Design review of the part built by this model. Coordinates are the model's own, in mm. A direction names the side the tool comes from. Coordinates: 2 decimals unless noted, no trailing zeros. Loops run counter-clockwise (first coordinate to the right, second up) from the corner with the lowest first, then second, coordinate; pieces in that order, holes last. Notation, with made-up numbers: M 37,-35 L 94,-35 A21 cw 94,-8 Z; hole C 10,47.25 d5. An arc over 180 degrees is marked long. Answer as a JSON object with one key per item and string values. Group by question number.
1. Draft analysis for pull direction Y (two halves, no side actions). For faces 1 (the cylindrical face through (11.27, 9.34, 7.3)), 2 (the cylindrical face through (1.7, 20.4, -2.2)), 3 (the cylindrical face through (4.054, 1.451, -3.168)), state which applies: +Y half, -Y half, draft (parallel to the pull), parting line (faces both ways), or undercut.
2. Insertion check: pin 1 (2 mm diameter, centred on x = 5.5, z = -2.5, fed in from -Y); pin 2 (1.8 mm diameter, centred on x = 10.5, y = 9.5, fed in from -Z); pin 3 (5.5 mm diameter, centred on x = 5.5, z = -3.5, fed in from +Y); pin 4 (1.5 mm diameter, centred on y = 3, z = 28, fed in from -X). Each pin has a flat end and moves straight along its axis. Give the tip position at first contact, or say it passes through.
3. Consider section C-C (x = 5.1). State the section outline as (y, z) points, then the cut area to 3 significant figures.
4. To check wall thickness, follow probe 1 along Z at (x, y) = (1.75, 19); probe 2 along Z at (x, y) = (1.75, 5.5); probe 3 along Y at (x, z) = (9.25, 13). State the ranges of each line that lie inside material, in increasing order.
5. Machinability: for faces 4 (the flat face through (6, 10, -0.9)), 5 (the cylindrical face through (0.63, 9.34, 7.3)), 6 (the flat face through (11.4, 0.5, 14.4)), 7 (the flat face through (6, 18.4, -2)), 8 (the cylindrical face through (0.66, 0.63, -0.46)), which of the approach directions +Z, -Z, +X, -X, +Y, -Y give a long, thin tool a straight path to every point of the face, cutting with its end or side? Answer none if there is none.
6. Consider section D-D (y = 5). State the section outline as (x, z) points, then the cut area to 3 significant figures.
7. Consider section B-B (y = 19). State the section outline as (x, z) points.
from build123d import *

# Parameters (mm, degrees)
SKETCH3_W           = 11.9
SKETCH3_H           = 10
BOSS_EXTRUDE1_DEPTH = 14.4
FILLET6_R           = 2.2
SKETCH6_W           = 11.9
SKETCH6_H           = 10
BOSS_EXTRUDE2_DEPTH = 8.9
SKETCH7_R           = 1.45
BOSS_EXTRUDE3_DEPTH = 9.5
SKETCH8_W           = 11.9
SKETCH8_H           = 18.4
BOSS_EXTRUDE4_DEPTH = 0.9
FILLET7_R           = 2.2
SKETCH9_R           = 4
BOSS_EXTRUDE6_DEPTH = 4.6
SKETCH10_W          = 11.9
SKETCH10_H          = 4.4
BOSS_EXTRUDE7_DEPTH = 4
SKETCH11_R          = 0.7
SKETCH11_R_2        = 0.702469816
SKETCH11_R_3        = 0.700963309
BOSS_EXTRUDE8_DEPTH = 4


with BuildPart() as part:
    # Sketch3 → Boss-Extrude1 (new body)
    with BuildSketch(Plane.XY):
        with Locations((5.95, 5)):
            Rectangle(SKETCH3_W, SKETCH3_H)
    extrude(amount=BOSS_EXTRUDE1_DEPTH)

    # Fillet6
    fillet6_edges = [part.edges().sort_by_distance(p)[0] for p in [
        (0, 10, 7.2),
        (11.9, 10, 7.2),
        (11.9, 0, 7.2),
        (0, 0, 7.2),
    ]]
    fillet(fillet6_edges, radius=FILLET6_R)

    # Sketch6 → Boss-Extrude2 (add)
    with BuildSketch(Plane.XY.offset(14.4)):
        with Locations((5.95, 5)):
            Rectangle(SKETCH6_W, SKETCH6_H)
    extrude(amount=BOSS_EXTRUDE2_DEPTH)

    # Sketch7 → Boss-Extrude3 (add)
    with BuildSketch(Plane.XY.offset(23.3)):
        with Locations((6.035152891, 5)):
            Circle(SKETCH7_R)
    extrude(amount=BOSS_EXTRUDE3_DEPTH)

    # Sketch8 → Boss-Extrude4 (add)
    with BuildSketch(Plane(origin=(0, 0, 0), x_dir=(-1, 0, 0), z_dir=(0, 0, -1))):
        with Locations((-5.95, 9.2)):
            Rectangle(SKETCH8_W, SKETCH8_H)
    extrude(amount=BOSS_EXTRUDE4_DEPTH)

    # Fillet7
    fillet7_edges = [part.edges().sort_by_distance(p)[0] for p in [
        (0, 0, -0.45),
        (11.9, 0, -0.45),
    ]]
    fillet(fillet7_edges, radius=FILLET7_R)

    # Sketch9 → Boss-Extrude6 (add)
    with BuildSketch(Plane(origin=(0, 0, -0.9), x_dir=(-1, 0, 0), z_dir=(0, 0, -1))):
        with Locations((-5.9, 5)):
            Circle(SKETCH9_R)
    extrude(amount=BOSS_EXTRUDE6_DEPTH)

    # Sketch10 → Boss-Extrude7 (add)
    with BuildSketch(Plane(origin=(0, 0, -0.9), x_dir=(-1, 0, 0), z_dir=(0, 0, -1))):
        with Locations((-5.95, 16.2)):
            Rectangle(SKETCH10_W, SKETCH10_H)
    extrude(amount=BOSS_EXTRUDE7_DEPTH)

    # Sketch11 → Boss-Extrude8 (add)
    with BuildSketch(Plane(origin=(0, 18.4, 0), x_dir=(1, 0, 0), z_dir=(0, 1, 0))):
        with Locations(Location((3.4, 2.9, 0), (0, 0, 90))):
            Circle(SKETCH11_R)
        with Locations(Location((5.1, 2.9, 0), (0, 0, 90))):
            Circle(SKETCH11_R)
        with Locations(Location((6.8, 2.9, 0), (0, 0, 90))):
            Circle(SKETCH11_R)
        with Locations(Location((8.5, 2.9, 0), (0, 0, 90))):
            Circle(SKETCH11_R_2)
        with Locations(Location((10.2, 2.9, 0), (0, 0, 90))):
            Circle(SKETCH11_R_3)
        with Locations(Location((1.7, 2.9, 0), (0, 0, 90))):
            Circle(SKETCH11_R)
    extrude(amount=BOSS_EXTRUDE8_DEPTH)


solid = part.part
Findings below:
{
 "1": {"face 1": "+Y half", "face 2": "draft", "face 3": "undercut"},
 "2": {"pin 1": "stops at y = 1", "pin 2": "stops at z = -0.9", "pin 3": "stops at y = 22.4", "pin 4": "stops at x = 5.3"},
 "3": {"outline": "M 0,-0.9 L 1.08,-0.9 L 1.08,-5.5 L 8.92,-5.5 L 8.92,-0.9 L 14,-0.9 L 14,-4.9 L 18.4,-4.9 L 18.4,-3.6 L 22.4,-3.6 L 22.4,-2.2 L 18.4,-2.2 L 18.4,0 L 10,0 L 10,23.3 L 6.11,23.3 L 6.11,32.8 L 3.89,32.8 L 3.89,23.3 L 0,23.3 Z", "area": "330 mm^2"},
 "4": {"probe 1": "z = -3.6 to -2.2", "probe 2": "z = -0.9 to 23.3", "probe 3": "y = 0 to 10"},
 "5": {"face 4": "-Z", "face 5": "-X, +Y", "face 6": "-Z, +X, -Y", "face 7": "+Y", "face 8": "-Z, -X, -Y"},
 "6": {"outline": "M 0,-0.9 L 1.9,-0.9 L 1.9,-5.5 L 9.9,-5.5 L 9.9,-0.9 L 11.9,-0.9 L 11.9,23.3 L 7.49,23.3 L 7.49,32.8 L 4.59,32.8 L 4.59,23.3 L 0,23.3 Z", "area": "352 mm^2"},
 "7": {"outline": "C 1.7,-2.9 d1.4; C 3.4,-2.9 d1.4; C 5.1,-2.9 d1.4; C 6.8,-2.9 d1.4; C 8.5,-2.9 d1.4; C 10.2,-2.9 d1.4"}
}
